```python
from build123d import *

# Parameters (mm, degrees)
F0_R     = 38.1
F0_R_2   = 30.704041
F1_DEPTH = 123.952
F2_R     = 5.08
F3_R     = 30.737392
F4_DEPTH = 6.35


with BuildPart() as f1:
    # F0 (on Front) → F1 (new body)
    with BuildSketch(Plane.XZ):
        Circle(F0_R)
        Circle(F0_R_2, mode=Mode.SUBTRACT)
    extrude(amount=F1_DEPTH)

    # F2
    f2_edges = [f1.edges().sort_by_distance(p)[0] for p in [
        (-38.1, -123.952, 0),
    ]]
    fillet(f2_edges, radius=F2_R)

    # F3 (on Front) → F4 (join)
    with BuildSketch(Plane.XZ):
        Circle(F3_R)
    extrude(amount=F4_DEPTH)


solid = f1.part
```
Model file for the job. Use its own axes, mm. A direction names the side the tool comes from. Round coordinates to 2 decimals unless told otherwise and drop trailing zeros. Loops run counter-clockwise (first coordinate to the right, second up) from the corner with the lowest first, then second, coordinate; pieces in that order, holes last. Notation, with made-up numbers: M 45,8.25 L 61,8.25 A35 ccw 61,40.25 Z; hole C 52.5,0.25 d6. An arc over 180 degrees is marked long. Put each result on its own line as item: value. Start each with the question number.
Item 1: Cut at C-C (y = -28). List the corners of the cut face in (x, z), then the cut area to 3 significant figures.
Item 2: 3-axis set-ups, long thin cutter, end or side, ignore diameter. For faces 4 (the face through (29.286, -64.328, 9.223)), 5 (the face through (22, -123.952, -22)): which of +Z, -Z, +X, -X, +Y, -Y reach the whole face in a straight line?
Item 3: Drop flat-ended pins along their axis: P1, Ø1, axis at x = -5, y = -71, coming from the +Z side; P2, Ø5, axis at x = -0.5, z = -23.5, coming from the -Y side; P3, Ø4, axis at y = -14.5, z = 11.5, coming from the -X side. Give the stop position or say it passes through.
Item 4: Mould opens along X. For faces 1 (the face through (0, -6.35, 0)), 2 (the face through (-1, 0, 1)), 3 (the face through (-30.235, -58.604, -23.183)) say: released by +X, released by -X, zero draft, split by the parting line, or undercut.
Item 5: Drill centre lines: line 1 along X through (y, z) = (-96.5, 0.5); line 2 along Y through (x, z) = (-11, -3). Where is each one in solid material? Low to high.
Item 6: Cut at A-A (z = 0). List the corners of the cut face in (x, y).
Item 7: Cut at B-B (x = 0). List the corners of the cut face in (y, z), then the cut area to 3 significant figures.
Answer block:
1. outline: C 0,0 d76.2; hole C 0,0 d61.41
1. area: 1,600 mm2
2. face 4: -Y
2. face 5: +Z, -Z, +X, -X, -Y
3. P1: z = 37.83
3. P2: y = -6.35
3. P3: x = -36.9
4. face 1: undercut
4. face 2: zero draft
4. face 3: split by the parting line
5. line 1: -38.1 to -30.7, 30.7 to 38.1
5. line 2: -6.35 to 0
6. outline: M -38.1,-118.87 A5.08 ccw -33.02,-123.95 L -30.7,-123.95 L -30.7,-6.35 L 30.7,-6.35 L 30.7,-123.95 L 33.02,-123.95 A5.08 ccw 38.1,-118.87 L 38.1,0 L -38.1,0 Z
7. outline: M -123.95,-33.02 A5.08 ccw -118.87,-38.1 L 0,-38.1 L 0,38.1 L -118.87,38.1 A5.08 ccw -123.95,33.02 L -123.95,30.7 L -6.35,30.7 L -6.35,-30.7 L -123.95,-30.7 Z
7. area: 2,210 mm2
